Verification items for this drawing (mm, ordinates from the low corner). A direction names the side the tool comes from. Round coordinates to 2 decimals unless told otherwise and drop trailing zeros. Loops run counter-clockwise (first coordinate to the right, second up) from the corner with the lowest first, then second, coordinate; pieces in that order, holes last. Notation, with made-up numbers: M 35,55 L 77,55 A28 cw 77,89 Z; hole C 34.25,0.25 d9. An arc over 180 degrees is marked long. Write item = value, one per line. Start each with the question number.
(1) Cross-section at A-A on x = 51. Record the boundary of the cut face in (y, z) (1 decimal).
(2) Mould release check, pull along Z, two halves, no side actions. Record for the marked faces 1, 2 and 3: pulls with the +Z half, pulls with the -Z half, needs draft (parallel to the pull), parting line crosses it, or undercut.
(3) Cross-section at B-B on z = 37.5. Record the boundary of the cut face in (x, y).
(4) Set-up check for the marked faces 4 and 5: record each of +Z, -Z, +X, -X, +Y, -Y from which the full face is reachable in a straight line by a thin tool's end or side.
(5) Scan lines: L1, parallel to X at y = 5, z = 45 (1 decimal); L2, parallel to Y at x = 27, z = 35.5; L3, parallel to X at y = 10, z = 42 (1 decimal). Record each from-to range of solid material in increasing order. Write a range as from..to.
(6) Cross-section at D-D on z = 70.5. Record the boundary of the cut face in (x, y), plus the area to 3 significant figures.
(7) Go/stop test with flat-tipped pins: P1, Ø1, axis at x = 78, y = 24, coming from the -Z side; P2, Ø1.5, axis at x = 92.5, z = 81, coming from the -Y side. Record where each tip stops, or that it passes through.
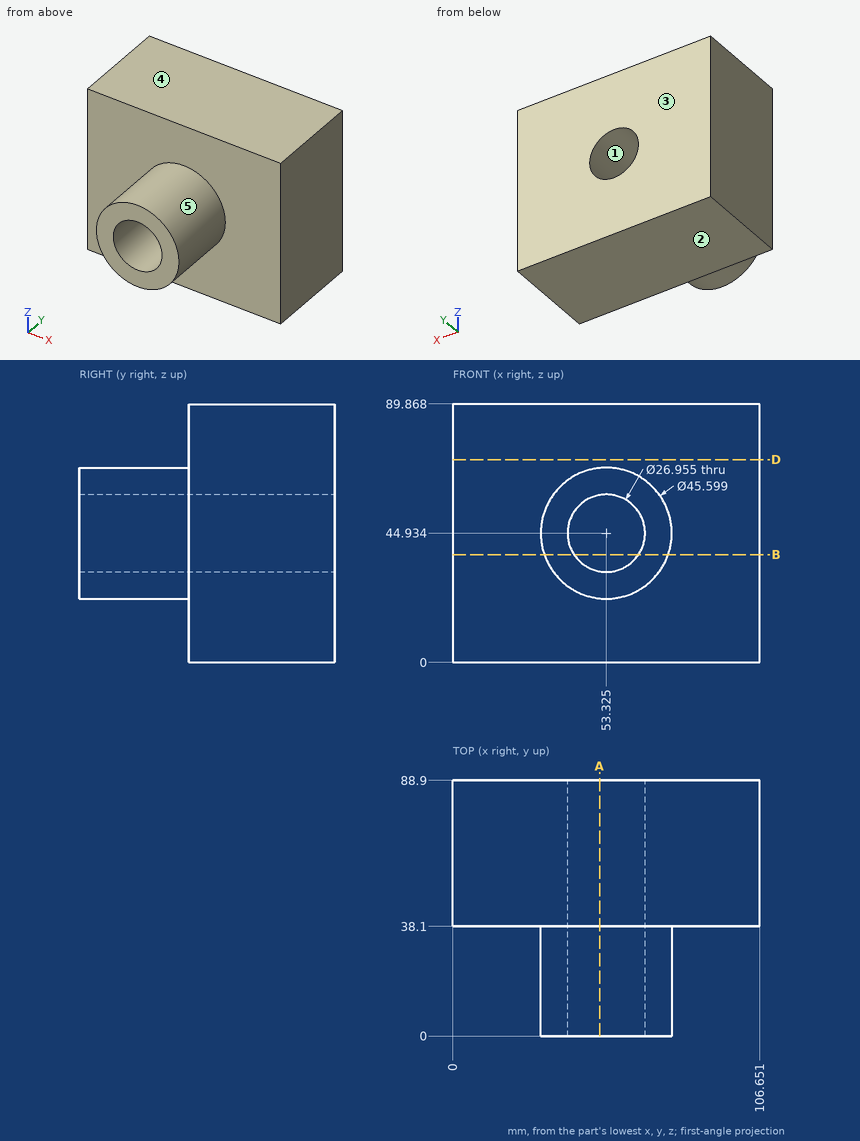
Result:
q1.outline = M 0,22.3 L 38.1,22.3 L 38.1,0 L 88.9,0 L 88.9,31.7 L 0,31.7 Z; M 0,58.2 L 88.9,58.2 L 88.9,89.9 L 38.1,89.9 L 38.1,67.6 L 0,67.6 Z
q2.face_1 = undercut
q2.face_2 = pulls with the -Z half
q2.face_3 = needs draft
q3.outline = M 0,38.1 L 31.77,38.1 L 31.77,0 L 42.08,0 L 42.08,88.9 L 0,88.9 Z; M 64.57,0 L 74.88,0 L 74.88,38.1 L 106.65,38.1 L 106.65,88.9 L 64.57,88.9 Z
q4.face_4 = +Z, +X, -X, +Y, -Y
q4.face_5 = -Y
q5.L1 = 30.5..39.8, 66.8..76.1
q5.L2 = 38.1..88.9
q5.L3 = 30.7..40.2, 66.5..75.9
q6.outline = M 0,38.1 L 106.65,38.1 L 106.65,88.9 L 0,88.9 Z
q6.area = 5,420 mm^2
q7.P1 = through
q7.P2 = 38.1
